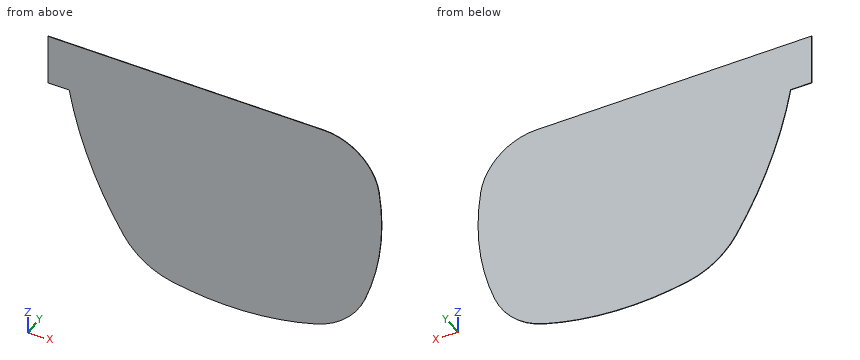
```python
from build123d import *

# Parameters (mm, degrees)
F1_DEPTH = 0.1


with BuildPart() as f1:
    # F0 (on Front) → F1 (new body)
    with BuildSketch(Plane.XZ):
        with BuildLine():
            Line((56, -2), (2, -2))
            Line((2, -2), (2, -12))
            Line((2, -12), (6.141136, -12))
            ThreePointArc((6.141136, -12), (10.197054, -26.094991), (16.819916, -39.181508))
            ThreePointArc((16.819916, -39.181508), (20.840447, -43.365146), (26.185783, -45.622329))
            ThreePointArc((26.185783, -45.622329), (40.395564, -46.669439), (54.431857, -44.220605))
            ThreePointArc((54.431857, -44.220605), (60.281606, -40.876074), (64.110749, -35.331427))
            ThreePointArc((64.110749, -35.331427), (67.098581, -23.520382), (66.873925, -11.339354))
            ThreePointArc((66.873925, -11.339354), (63.167039, -4.655328), (56, -2))
        make_face()
    extrude(amount=-F1_DEPTH)


solid = f1.part
```
Work out the finished part from the listing and answer in its coordinate system (mm). Coordinates: 2 decimals unless noted, no trailing zeros. Loops run counter-clockwise (first coordinate to the right, second up) from the corner with the lowest first, then second, coordinate; pieces in that order, holes last. Notation, with made-up numbers: (-18, 68.5) - (27, 68.5) arc R15 ccw to (27, 91.5) - close; hole circle Ø8 at (-2, 64.25). An arc over 180 degrees is marked (long way). Use a Markdown table: item, result.
Item 1: Consider probe 1 along X at (y, z) = (0.05, -7.5); probe 2 along X at (y, z) = (0.05, -25.5); probe 3 along Z at (x, y) = (47.5, 0.05). Determine where each line is inside the solid, lowest interval first. Write a range as from..to.
Evaluation:
| item | result |
|---|---|
| probe 1 | x = 2..65.53 |
| probe 2 | x = 9.97..66.83 |
| probe 3 | z = -45.88..-2 |
Item 2: Find section A-A, the plane z = -24. Determine the outline of the cut face in (x, y).
Evaluation:
| item | result |
|---|---|
| outline | (9.41, 0) - (67.04, 0) - (67.04, 0.1) - (9.41, 0.1) - close |
Item 3: Find section B-B, the plane x = 9. Determine the outline of the cut face in (y, z).
Evaluation:
| item | result |
|---|---|
| outline | (0, -22.84) - (0.1, -22.84) - (0.1, -2) - (0, -2) - close |
Item 4: Given pin 1 Ø6 at (x, z) = (9, -31.5) entering from -Y, flat-ended and moving along its own axis, determine where the tip first touches the part or whether it passes through.
Evaluation:
| item | result |
|---|---|
| pin 1 | passes through |
